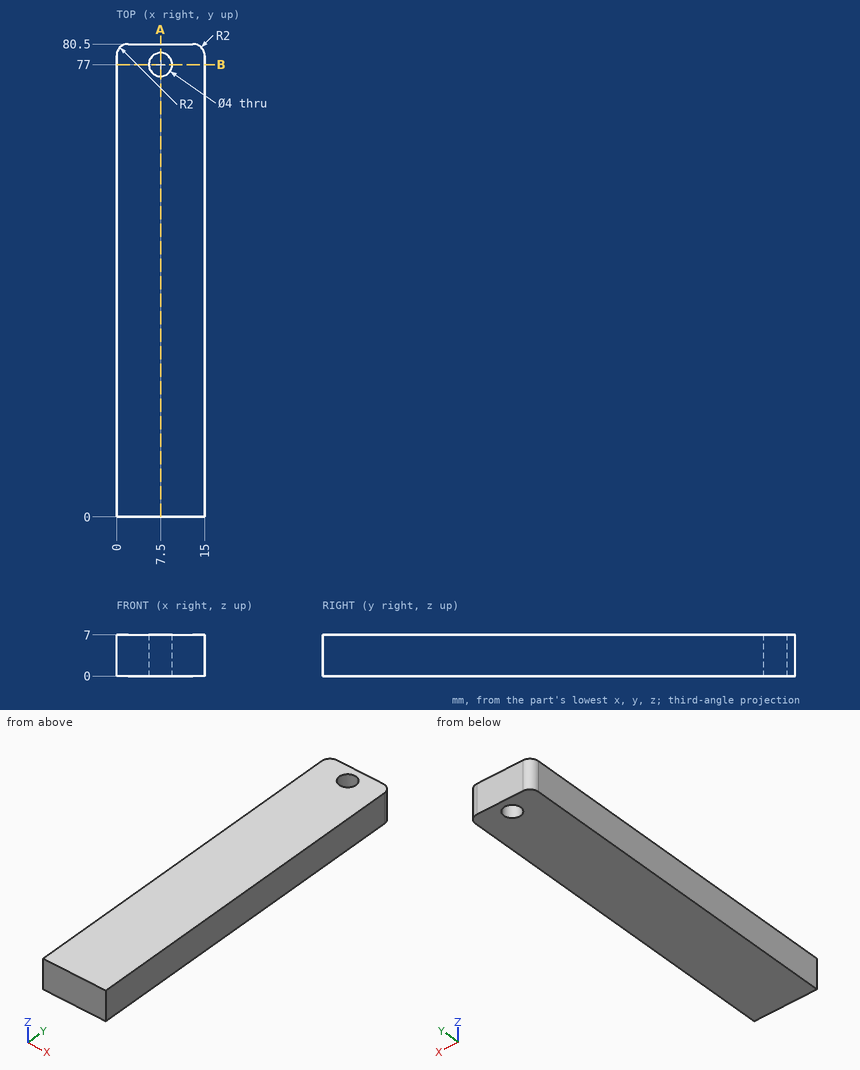
Could you check a few things on this drawing? It's one solid part, dimensions in mm from its lowest x, y, z. Coordinates: 2 decimals unless noted, no trailing zeros. Write each loop counter-clockwise with the first axis right and the second up, starting at its lowest first coordinate (ties: lowest second). Pieces come first, ordered by that corner, then holes.
1) If we section it at B-B (y = 77): List the corners of the cut face in (x, z) for me.
Filled in:
outline: (0, 0) - (5.5, 0) - (5.5, 7) - (0, 7) - close; (9.5, 0) - (15, 0) - (15, 7) - (9.5, 7) - close
2) If we section it at A-A (x = 7.5): List the corners of the cut face in (y, z) for me.
Filled in:
outline: (0, 0) - (75, 0) - (75, 7) - (0, 7) - close; (79, 0) - (80.5, 0) - (80.5, 7) - (79, 7) - close
3) If I drill on line 1 (Y direction, x = 7.75, z = 1.25); line 2 (Y direction, x = 7, z = 2.75); line 3 (Y direction, x = 1.5, z = 2.25), over which ranges is the centre line in solid material (lowest first)?
Filled in:
line 1: y = 0 to 75.02, 78.98 to 80.5
line 2: y = 0 to 75.06, 78.94 to 80.5
line 3: y = 0 to 80.44
